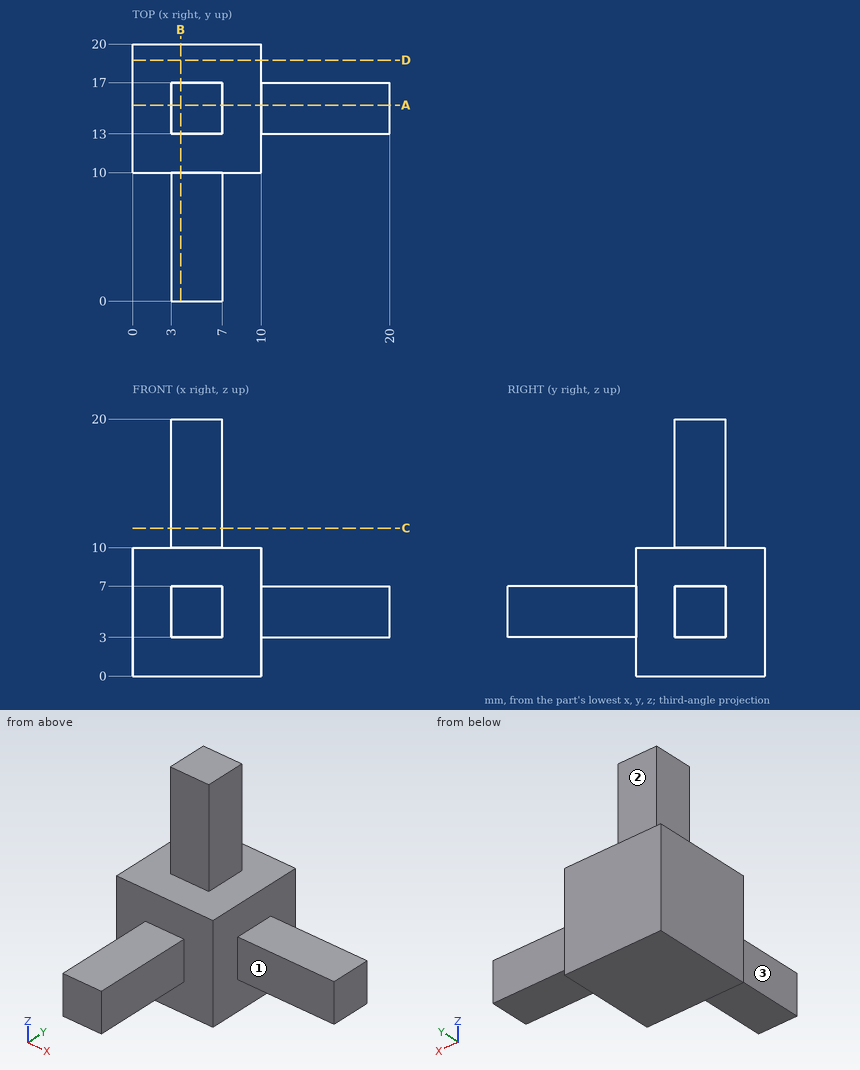
Here's the drawing with two shaded views (mm, measured from the low corner). I have some questions. A direction names the side the tool comes from. Coordinates: 2 decimals unless noted, no trailing zeros. Order: outer loops, then holes, each group sorted by start corner. A loop starts at its lowest first (then second) coordinate and runs counter-clockwise, first axis right, second up. Notation, with made-up numbers: M 80,77 L 96,77 A20 cw 96,92 Z; hole C -38.75,68.25 d11. An arc over 180 degrees is marked long. Write item = value, one per line.
(1) Suppose I cut it at C-C on z = 11.5. Please give me the cut outline in (x, y).
Results are:
outline = M 3,13 L 7,13 L 7,17 L 3,17 Z
(2) Suppose I cut it at B-B on x = 3.75. Please give me the cut outline in (y, z), plus the area to 3 significant figures.
Results are:
outline = M 0,3 L 10,3 L 10,0 L 20,0 L 20,10 L 17,10 L 17,20 L 13,20 L 13,10 L 10,10 L 10,7 L 0,7 Z
area = 180 mm2
(3) Suppose I cut it at A-A on y = 15.25. Please give me the cut outline in (x, z).
Results are:
outline = M 0,0 L 10,0 L 10,3 L 20,3 L 20,7 L 10,7 L 10,10 L 7,10 L 7,20 L 3,20 L 3,10 L 0,10 Z
(4) I need wall thicknesses on line 1 along Y through (x, z) = (2.25, 3); line 2 along X through (y, z) = (16.75, 11); line 3 along X through (y, z) = (12, 5.5). Which ranges of each line are inside material? Lowest first, please. Write a range as [from, to].
Results are:
line_1 = [10, 20]
line_2 = [3, 7]
line_3 = [0, 10]
(5) For pin 1 Ø4.5 at (x, z) = (13, 5) entering from -Y; pin 2 Ø1 at (y, z) = (5, 5.5) entering from +X; pin 3 Ø4.5 at (x, y) = (16, 15.5) entering from +Z; pin 4 Ø6 at (x, y) = (14.5, 8) entering from -Z, each with a flat end and sliding along its axis, tell me the tip position at first contact or that it passes through.
Results are:
pin_1 = 13
pin_2 = 7
pin_3 = 7
pin_4 = through
(6) Suppose I cut it at D-D on y = 18.75. Please give me the cut outline in (x, z).
Results are:
outline = M 0,0 L 10,0 L 10,10 L 0,10 Z
(7) For the marked faces 1, 2 and 3, which set-ups out of +Z, -Z, +X, -X, +Y, -Y let a thin tool reach every point of the face, with its end or its side?
Results are:
face_1 = +Z, -Z, +X, -Y
face_2 = +Z, +X, -X, +Y
face_3 = +Z, -Z, -X, -Y
